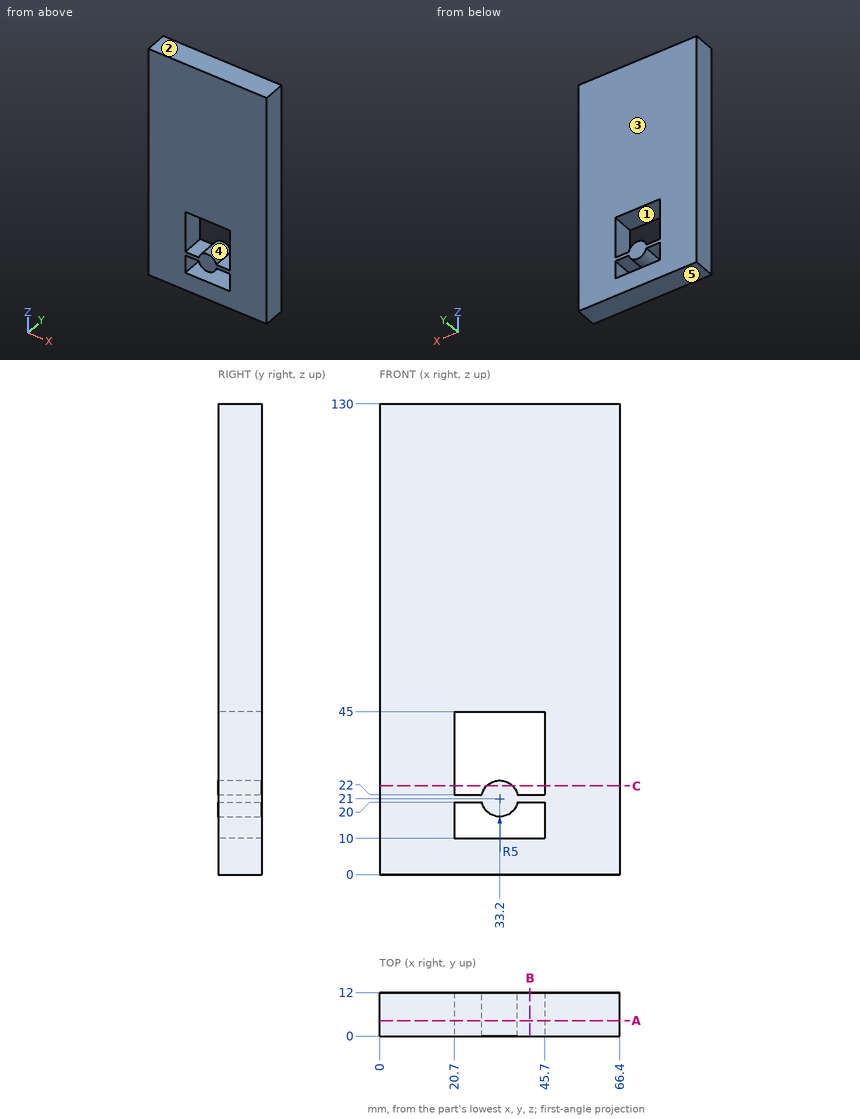
Design review of the part shown in the three views and the two pictorial views. Dimensions are in mm from the part's minimum x, y and z. A direction names the side the tool comes from. Round coordinates to 2 decimals unless told otherwise and drop trailing zeros. Write each loop counter-clockwise with the first axis right and the second up, starting at its lowest first coordinate (ties: lowest second). Pieces come first, ordered by that corner, then holes. Notation, with made-up numbers: M -10,-4 L 44,-4 A18 cw 44,29 Z; hole C 39.5,-3.75 d2. An arc over 180 degrees is marked long. One line per item, written item: value. Start each with the question number.
1. Take a section at B-B on x = 41.5. State the section outline as (y, z) points.
2. Take a section at C-C on z = 24.5. State the section outline as (x, y) points, then the cut area to 3 significant figures.
3. Draft analysis for pull direction Z (two halves, no side actions). For the marked faces 1, 2 and 3, state which applies: pulls with the +Z half, pulls with the -Z half, needs draft (parallel to the pull), parting line crosses it, or undercut.
4. Take a section at A-A on y = 4.25. State the section outline as (x, z) points, then the cut area to 3 significant figures.
5. To check wall thickness, follow probe 1 along Z at (x, y) = (44, 5.5); probe 2 along X at (y, z) = (9.75, 11); probe 3 along Z at (x, y) = (35, 6.25). State the ranges of each line that lie inside material, in increasing order. Write a range as from..to.
6. For the marked faces 4 and 5, list the 3-axis set-ups (+Z, -Z, +X, -X, +Y, -Y) from which the entire face can be reached by the end or side of a thin tool; tool diameter is ignored.
Computed:
1. outline: M 0,0 L 12,0 L 12,10 L 0,10 Z; M 0,20 L 12,20 L 12,22 L 0,22 Z; M 0,45 L 12,45 L 12,130 L 0,130 Z
2. outline: M 0,0 L 20.7,0 L 20.7,12 L 0,12 Z; M 29.63,0 L 36.77,0 L 36.77,12 L 29.63,12 Z; M 45.7,0 L 66.4,0 L 66.4,12 L 45.7,12 Z
2. area: 582 mm²
3. face 1: undercut
3. face 2: pulls with the +Z half
3. face 3: needs draft
4. outline: M 0,0 L 66.4,0 L 66.4,130 L 0,130 Z; hole M 20.7,10 L 45.7,10 L 45.7,20 L 38.1,20 A5 cw 28.3,20 L 20.7,20 Z; hole M 20.7,22 L 28.3,22 A5 cw 38.1,22 L 45.7,22 L 45.7,45 L 20.7,45 Z
4. area: 7,870 mm²
5. probe 1: z = 0..10, 20..22, 45..130
5. probe 2: x = 0..20.7, 45.7..66.4
5. probe 3: z = 0..10, 16.34..25.66, 45..130
6. face 4: +Y, -Y
6. face 5: -Z, +X, -X, +Y, -Y
